Source: CAD feature listing. Evaluate the final solid. Frame: model axes, mm. A direction names the side the tool comes from. Coordinates: 2 decimals unless noted, no trailing zeros. Order: outer loops, then holes, each group sorted by start corner. A loop starts at its lowest first (then second) coordinate and runs counter-clockwise, first axis right, second up. Notation, with made-up numbers: (37.5, 43.5) - (77.5, 43.5) arc R33 ccw to (77.5, 77.5) - close; hole circle Ø8 at (57.5, -31). An arc over 180 degrees is marked (long way). One line per question, with ' | ' between items.
from build123d import *

# Parameters (mm, degrees)
BOSS_EXTRUDE1_DEPTH = 6
SKETCH2_W           = 66
SKETCH2_H           = 275
BOSS_EXTRUDE2_DEPTH = 6
SKETCH3_R           = 10
CUT_EXTRUDE1_DEPTH  = 6


with BuildPart() as part:
    # Sketch1 → Boss-Extrude1 (new body)
    with BuildSketch(Plane.XY):
        Polygon((23, 255), (23, 0), (43, 0), (43, 275), (-23, 275), (-23, 255), align=None)
    extrude(amount=-BOSS_EXTRUDE1_DEPTH)

    # Sketch2 → Boss-Extrude2 (add)
    with BuildSketch(Plane.XY):
        with Locations((10, 137.5)):
            Rectangle(SKETCH2_W, SKETCH2_H)
    extrude(amount=BOSS_EXTRUDE2_DEPTH)

    # Sketch3 → Cut-Extrude1 (cut)
    with BuildSketch(Plane(origin=(0, 0, -6), x_dir=(-1, 0, 0), z_dir=(0, 0, -1))):
        with Locations((-23, 255)):
            Circle(SKETCH3_R)
    extrude(amount=-CUT_EXTRUDE1_DEPTH, mode=Mode.SUBTRACT)


solid = part.part
(1) Material intervals for L1, parallel to Y at x = 28.5, z = -5; L2, parallel to Y at x = 30, z = -3.75; L3, parallel to X at y = 19.5, z = -5, sorted ascending. Write a range as from..to.
Taken from the geometry:
L1: y = 0..246.65, 263.35..275 | L2: y = 0..247.86, 262.14..275 | L3: x = 23..43
(2) Pin query (flat end, axial travel): P1, Ø5, axis at x = 3.5, z = -4.5, coming from the -Y side; P2, Ø3, axis at y = 95.5, z = -2, coming from the -X side; P3, Ø1, axis at x = 14.5, y = 202, coming from the -Z side. Return the tip coordinate at first contact, or that it passes through.
Taken from the geometry:
P1: stops at y = 255 | P2: stops at x = 23 | P3: stops at z = 0
(3) Set-up query: faces 1 (the flat face through (-5, 255, -3)), 2 (the cylindrical face through (29.834, 262.3, -3.042)), 3 (the flat face through (43, 136, 0)). Return all of +Z, -Z, +X, -X, +Y, -Y with unobstructed straight access to the full face (end or side cutting, diameter ignored); none if empty.
Taken from the geometry:
face 1: -Z, -X, -Y | face 2: -Z | face 3: +Z, -Z, +X, +Y, -Y
(4) Cut plane B-B (x = -14). Return the cut outline in (y, z).
Taken from the geometry:
outline: (0, 0) - (255, 0) - (255, -6) - (275, -6) - (275, 6) - (0, 6) - close
(5) Cut plane A-A (y = 146). Return the cut outline in (x, z).
Taken from the geometry:
outline: (-23, 0) - (23, 0) - (23, -6) - (43, -6) - (43, 6) - (-23, 6) - close
